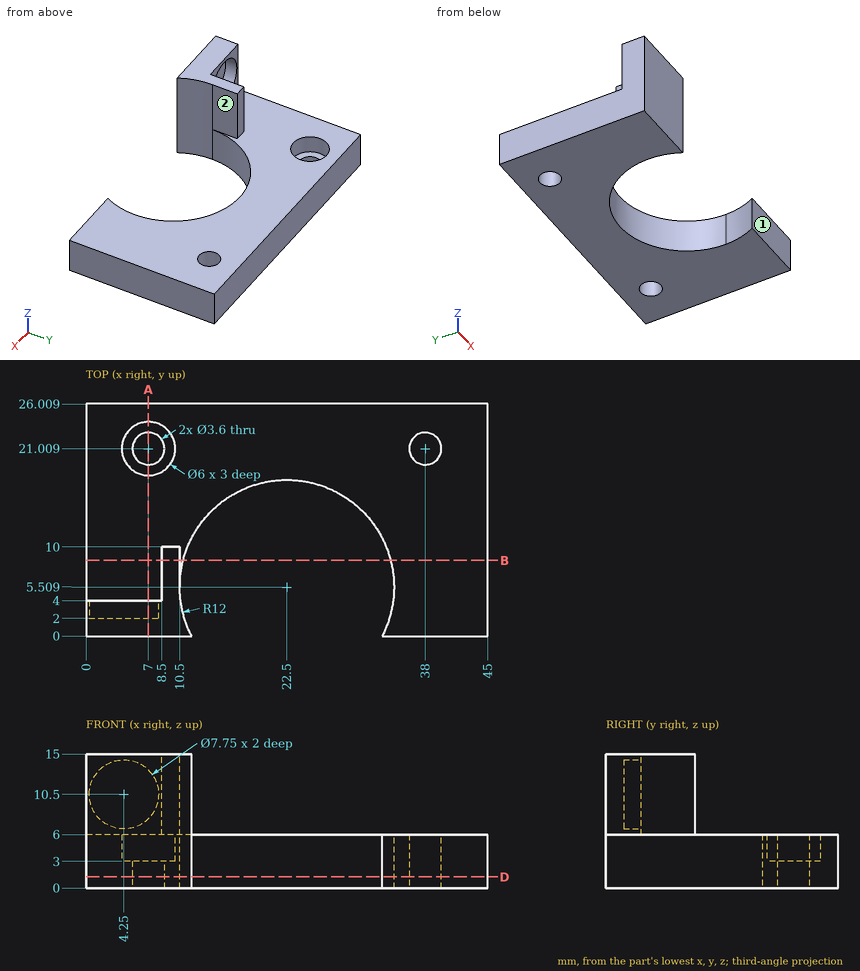
Study the drawing (mm; zero at the part's minimum x, y, z) and answer. A direction names the side the tool comes from. Coordinates: 2 decimals unless noted, no trailing zeros. Write each loop counter-clockwise with the first axis right and the second up, starting at its lowest first coordinate (ties: lowest second). Pieces come first, ordered by that corner, then holes. Notation, with made-up numbers: (73.5, 84.25) - (90.5, 84.25) arc R18 ccw to (90.5, 115.25) - close; hole circle Ø4 at (62.5, 70). An arc over 180 degrees is marked (long way). Answer as a JSON object with one key per item and string values. Group by question number.
1. Which of the six approach directions +Z, -Z, +X, -X, +Y, -Y give full straight-line access (tool end or side, diameter ignored) to the marked faces 1 and 2?
2. A cutting plane is placed at D-D (z = 1.25). Determine the outline of the cut face in (x, y).
3. A cutting plane is placed at B-B (y = 8.5). Determine the outline of the cut face in (x, z), plus the area to 3 significant figures.
4. Consider L1, parallel to Y at x = 38, z = 1.3; L2, parallel to X at y = 19.5, z = 4.75; L3, parallel to Y at x = 7, z = 4.25. Determine where each line is inside the solid, lowest interval first. Write a range as [from, to].
5. Each of these flat-tipped pins is pushed along its axis until it touches: P1, Ø8, axis at x = 40, y = 3.5, coming from the +Z side; P2, Ø1.8, axis at y = 6.5, z = 10, coming from the -X side; P3, Ø7, axis at x = 4.25, z = 10.5, coming from the +Y side; P4, Ø1, axis at x = 13.5, z = 12, coming from the -Y side. Where does it stop, or does it pass through?
6. A cutting plane is placed at A-A (x = 7). Determine the outline of the cut face in (y, z).
Worked out:
{
 "1": {"face 1": "+Z, -Z, +X, -X, -Y", "face 2": "+Z, +X, +Y"},
 "2": {"outline": "(0, 0) - (11.84, 0) arc R12 cw (long way) to (33.16, 0) - (45, 0) - (45, 26.01) - (0, 26.01) - close; hole circle Ø3.6 at (7, 21.01); hole circle Ø3.6 at (38, 21.01)"},
 "3": {"outline": "(0, 0) - (10.88, 0) - (10.88, 6) - (10.5, 6) - (10.5, 15) - (8.5, 15) - (8.5, 6) - (0, 6) - close; (34.12, 0) - (45, 0) - (45, 6) - (34.12, 6) - close", "area": "149 mm²"},
 "4": {"L1": "y = [0, 19.21], [22.81, 26.01]", "L2": "x = [0, 4.41], [9.59, 37.02], [38.98, 45]", "L3": "y = [0, 18.01], [24.01, 26.01]"},
 "5": {"P1": "stops at z = 6", "P2": "stops at x = 8.5", "P3": "stops at y = 2", "P4": "passes through"},
 "6": {"outline": "(0, 0) - (19.21, 0) - (19.21, 3) - (18.01, 3) - (18.01, 6) - (4, 6) - (4, 7.77) - (2, 7.77) - (2, 13.23) - (4, 13.23) - (4, 15) - (0, 15) - close; (22.81, 0) - (26.01, 0) - (26.01, 6) - (24.01, 6) - (24.01, 3) - (22.81, 3) - close"}
}
